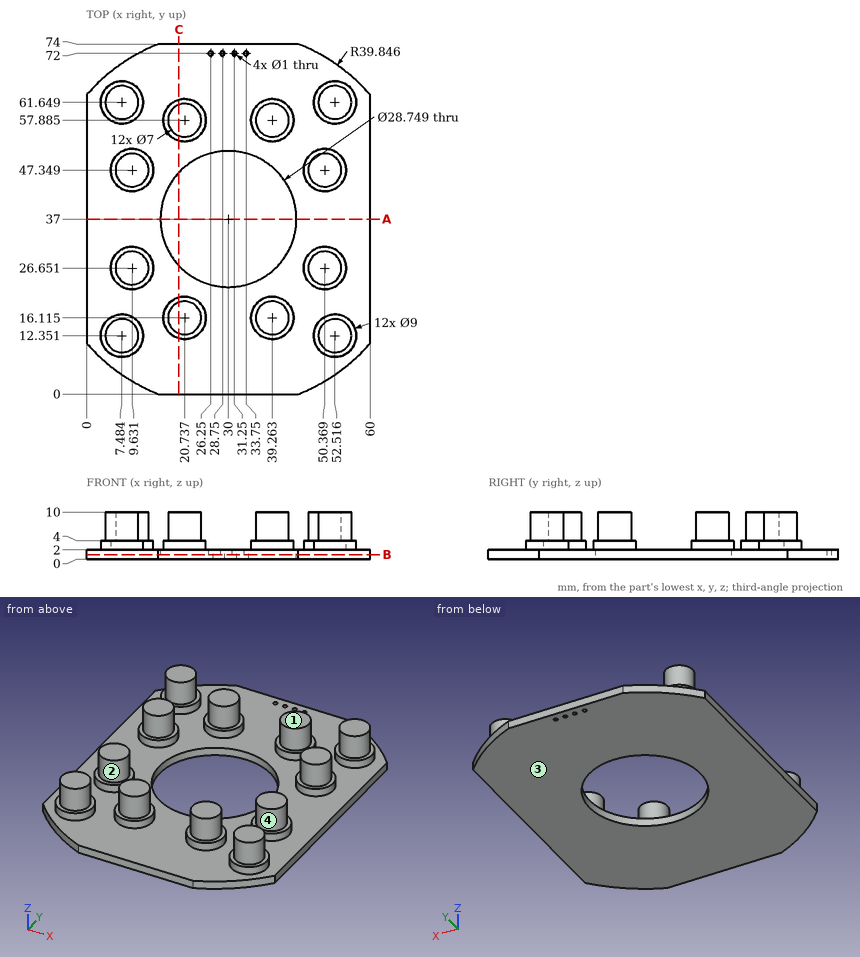
Study the drawing (mm; zero at the part's minimum x, y, z) and answer. A direction names the side the tool comes from. Give positions to 0.01 mm unless a question says otherwise; leave off trailing zeros. Write each loop counter-clockwise with the first axis right and the second up, starting at its lowest first coordinate (ties: lowest second). Pieces come first, ordered by that corner, then holes. Notation, with made-up numbers: (-21, 31.25) -> (-4, 31.25) arc R36 cw to (-4, 65.25) -> close; hole circle Ø10 at (25.5, 23.5). An arc over 180 degrees is marked (long way). Answer as a JSON object with one key per item and string values. Group by question number.
1) Each of these flat-tipped pins is pushed along its axis until it touches: P1, Ø1, axis at x = 43, z = 3.5, coming from the -Y side; P2, Ø23, axis at x = 30, y = 37, coming from the +Z side; P3, Ø3, axis at y = 66, z = 5, coming from the +X side (1 decimal); P4, Ø1, axis at x = 19, y = 21.5, coming from the +Z side. Where does it stop, or does it pass through?
2) Find section C-C (x = 19.5). Write down the section's boundary in (y, z).
3) The mould has two halves that part along Y. Classify the marked faces 1 and 2: +Y half, -Y half, draft (parallel to the pull), parting line (faces both ways), or undercut.
4) A tool of negligible diameter and unlimited length cuts with its end or side. For the marked faces 3 and 4, from which of +Z, -Z, +X, -X, +Y, -Y can it reach the whole face along a straight path? Write none if from no direction.
5) Find section B-B (z = 1). Count the separate pieces of the cut face and the enclosed holes in it, and give its area (4 significant figures).
6) Find section A-A (y = 37). Write down the section's boundary in (x, z) (1 decimal).
7) Consider L1, parallel to Y at x = 28.75, z = 0.5; L2, parallel to Z at x = 55, y = 40; L3, parallel to Y at x = 50, z = 5 (1 decimal). Determine where each line is inside the solid, lowest interval first. Write a range as from..to.
Values follow:
{
 "1": {"P1": "stops at y = 12.99", "P2": "passes through", "P3": "stops at x = 55.6", "P4": "stops at z = 2"},
 "2": {"outline": "(0, 0) -> (27.18, 0) -> (27.18, 2) -> (20.44, 2) -> (20.44, 4) -> (19.39, 4) -> (19.39, 10) -> (12.84, 10) -> (12.84, 4) -> (11.79, 4) -> (11.79, 2) -> (0, 2) -> close; (46.82, 0) -> (74, 0) -> (74, 2) -> (62.21, 2) -> (62.21, 4) -> (61.16, 4) -> (61.16, 10) -> (54.61, 10) -> (54.61, 4) -> (53.56, 4) -> (53.56, 2) -> (46.82, 2) -> close"},
 "3": {"face 1": "draft", "face 2": "undercut"},
 "4": {"face 3": "-Z, +X, -X, +Y, -Y", "face 4": "+Z"},
 "5": {"separate pieces": "1", "enclosed holes": "5", "area": "3,515 mm2"},
 "6": {"outline": "(0, 0) -> (15.6, 0) -> (15.6, 2) -> (0, 2) -> close; (44.4, 0) -> (60, 0) -> (60, 2) -> (44.4, 2) -> close"},
 "7": {"L1": "y = 0..22.68, 51.32..71.5, 72.5..74", "L2": "z = 0..2", "L3": "y = 9.9..14.8, 23.2..30.1, 43.9..50.8, 59.2..64.1"}
}
